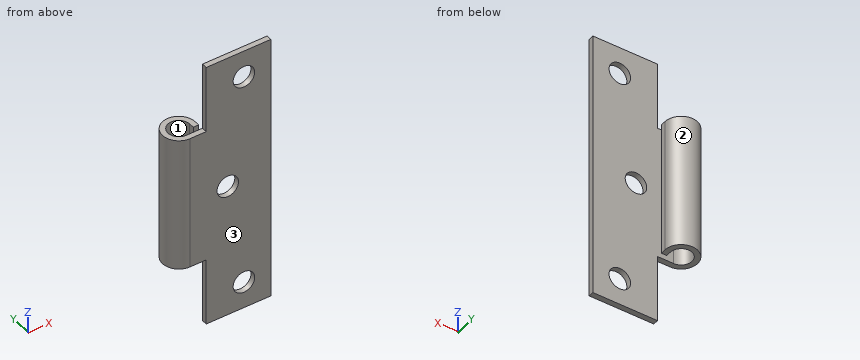
from build123d import *

# Parameters (mm, degrees)
F1_DEPTH = 50
F3_D     = 4
F3_DEPTH = 10
F2_W     = 8
F2_H     = 12.5
F4_DEPTH = 25


with BuildPart() as f1:
    # F0 (on Top) → F1 (new body)
    with BuildSketch(Plane.XY):
        with BuildLine():
            Line((15, 1), (0, 1))
            ThreePointArc((0, 1), (-1.414214, 4.414214), (2, 3))
            Line((2, 3), (2, 2))
            Line((2, 2), (3, 2))
            Line((3, 2), (3, 3))
            ThreePointArc((3, 3), (-2.12132, 5.12132), (0, 0))
            Line((0, 0), (15, 0))
            Line((15, 0), (15, 1))
        make_face()
    extrude(amount=F1_DEPTH)

    # F3
    with Locations(Plane.XZ):
        with Locations((10, 45), (7, 25), (10, 5)):
            Hole(F3_D / 2, depth=F3_DEPTH)

    # F2 (on Front) → F4 (cut)
    with BuildSketch(Plane.XZ):
        with Locations((-1, 43.75)):
            Rectangle(F2_W, F2_H)
        with Locations((-1, 6.25)):
            Rectangle(F2_W, F2_H)
    extrude(amount=-F4_DEPTH, mode=Mode.SUBTRACT)


solid = f1.part
Source: CAD feature listing. Evaluate the final solid. Frame: model axes, mm. Face numbers are marked on the shaded views. Give positions to 0.01 mm unless a question says otherwise; leave off trailing zeros. Write each loop counter-clockwise with the first axis right and the second up, starting at its lowest first coordinate (ties: lowest second). Pieces come first, ordered by that corner, then holes. Notation, with made-up numbers: (82.5, -31.75) - (108.5, -31.75) arc R21 cw to (108.5, -16.75) - close; hole circle Ø6 at (21.25, 45.25). An arc over 180 degrees is marked (long way). Write item = value, one per line. Start each with the question number.
Q1. Cut plane C-C, the plane x = 10. Return loops of the section in (y, z), then the cut area to 3 significant figures.
Q2. Draft query along X for the marked faces 1, 2 and 3. Return one class per face: +X half, -X half, draft (parallel to the pull), parting line (faces both ways), or undercut.
Q3. Pin query (flat end, axial travel): pin 1 Ø3 at (x, y) = (1.5, 2) entering from -Z; pin 2 Ø1.1 at (y, z) = (0.5, 4) entering from -X; pin 3 Ø3 at (x, y) = (-0.5, 2.5) entering from +Z; pin 4 Ø3 at (x, z) = (7, 25) entering from +Y. Return the tip coordinate at first contact, or that it passes through.
Q4. Cut plane B-B, the plane x = 7. Return loops of the section in (y, z).
Q5. Material intervals for probe 1 along Z at (x, y) = (10, 0.5); probe 2 along Z at (x, y) = (7, 0.35); probe 3 along X at (y, z) = (3.05, 33.5), sorted ascending.
Q6. Cut plane A-A, the plane z = 5. Return loops of the section in (x, y), then the cut area to 3 significant figures.
Q7. Cut plane D-D, the plane z = 25. Return loops of the section in (x, y).
Computed values:
q1.outline = (0, 0) - (1, 0) - (1, 3) - (0, 3) - close; (0, 7) - (1, 7) - (1, 43) - (0, 43) - close; (0, 47) - (1, 47) - (1, 50) - (0, 50) - close
q1.area = 42.0 mm²
q2.face_1 = undercut
q2.face_2 = parting line
q2.face_3 = draft
q3.pin_1 = 12.5
q3.pin_2 = 3
q3.pin_3 = 37.5
q3.pin_4 = through
q4.outline = (0, 0) - (1, 0) - (1, 23) - (0, 23) - close; (0, 27) - (1, 27) - (1, 50) - (0, 50) - close
q5.probe_1 = 0 to 3, 7 to 43, 47 to 50
q5.probe_2 = 0 to 23, 27 to 50
q5.probe_3 = -3 to -2, 2 to 3
q6.outline = (3, 0) - (8, 0) - (8, 1) - (3, 1) - close; (12, 0) - (15, 0) - (15, 1) - (12, 1) - close
q6.area = 8.00 mm²
q7.outline = (0, 0) - (5, 0) - (5, 1) - (0, 1) arc R2 cw (long way) to (2, 3) - (2, 2) - (3, 2) - (3, 3) arc R3 ccw (long way) to start; (9, 0) - (15, 0) - (15, 1) - (9, 1) - close
